Model file for the job. Use its own axes, mm. Round coordinates to 2 decimals unless told otherwise and drop trailing zeros. Loops run counter-clockwise (first coordinate to the right, second up) from the corner with the lowest first, then second, coordinate; pieces in that order, holes last.
from build123d import *

# Parameters (mm, degrees)
SKETCH1_W           = 60
SKETCH1_H           = 170
BOSS_EXTRUDE1_DEPTH = 0.5
SKETCH2_W           = 34
SKETCH2_H           = 55
CUT_EXTRUDE1_DEPTH  = 10


with BuildPart() as part:
    # Sketch1 → Boss-Extrude1 (new body)
    with BuildSketch(Plane(origin=(0, 0, 0), x_dir=(1, 0, 0), z_dir=(0, 1, 0))):
        Rectangle(SKETCH1_W, SKETCH1_H)
    extrude(amount=BOSS_EXTRUDE1_DEPTH)

    # Sketch2 → Cut-Extrude1 (cut)
    with BuildSketch(Plane.XZ):
        with Locations((0, 7.5)):
            Rectangle(SKETCH2_W, SKETCH2_H)
    extrude(amount=-CUT_EXTRUDE1_DEPTH, mode=Mode.SUBTRACT)


solid = part.part
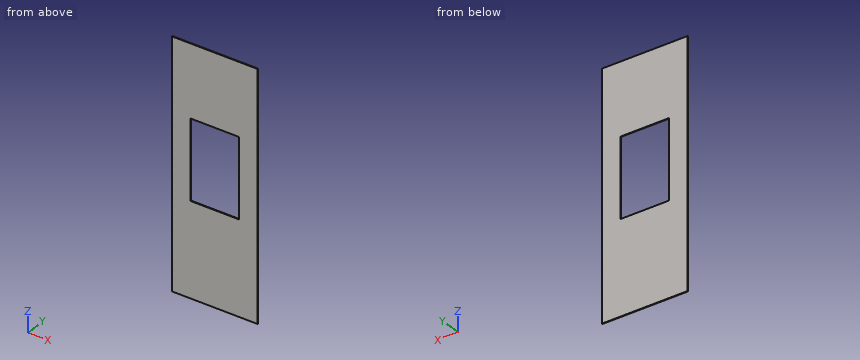
Q1. Slice it at C-C on y = 0.25. Give the cut face in (x, z).
Q2. Probe line 1 (Z direction, x = 13, y = 0.35); line 2 (X direction, y = 0.45, z = 28.5). List the from-to ranges inside material, lowest first.
Q3. Slice it at B-B on z = 12. Give the cut face in (x, y), plus the area to 3 significant figures.
Q4. Slice it at A-A on x = -15. Give the cut face in (y, z).
Reply:
1. outline: (-30, -85) - (30, -85) - (30, 85) - (-30, 85) - close; hole (-17, -20) - (17, -20) - (17, 35) - (-17, 35) - close
2. line 1: z = -85 to -20, 35 to 85
2. line 2: x = -30 to -17, 17 to 30
3. outline: (-30, 0) - (-17, 0) - (-17, 0.5) - (-30, 0.5) - close; (17, 0) - (30, 0) - (30, 0.5) - (17, 0.5) - close
3. area: 13.0 mm2
4. outline: (0, -85) - (0.5, -85) - (0.5, -20) - (0, -20) - close; (0, 35) - (0.5, 35) - (0.5, 85) - (0, 85) - close
